```python
from build123d import *

# Parameters (mm, degrees)
F0_W     = 600
F0_H     = 700
F1_DEPTH = 540
F2_W     = 600
F2_H     = 560
F3_DEPTH = 300
F4_W     = 200
F4_H     = 140
F5_DEPTH = 200
F6_W     = 250
F6_H     = 600
F7_DEPTH = 140
F8_R     = 75
F9_DEPTH = 100.001


with BuildPart() as f1:
    # F0 (on Front) → F1 (new body)
    with BuildSketch(Plane.XZ):
        Rectangle(F0_W, F0_H)
    extrude(amount=F1_DEPTH)

    # F2 (on face) → F3 (cut)
    with BuildSketch(Plane.XZ.offset(540)):
        with Locations((0, 70)):
            Rectangle(F2_W, F2_H)
    extrude(amount=-F3_DEPTH, mode=Mode.SUBTRACT)

    # F4 (on face) → F5 (cut)
    with BuildSketch(Plane.XZ.offset(540)):
        with Locations((0, -280)):
            Rectangle(F4_W, F4_H)
    extrude(amount=-F5_DEPTH, mode=Mode.SUBTRACT)

    # F6 (on face) → F7 (cut)
    with BuildSketch(Plane.XZ.offset(240)):
        with BuildLine():
            ThreePointArc((-125, 50), (0, -75), (125, 50))
            Line((125, 50), (-125, 50))
        make_face()
        with Locations((0, 350)):
            Rectangle(F6_W, F6_H)
    extrude(amount=-F7_DEPTH, mode=Mode.SUBTRACT)

    # F8 (on face) → F9 (cut, through all)
    with BuildSketch(Plane.XZ.offset(100)):
        with Locations((0, 100)):
            Circle(F8_R)
    extrude(amount=-F9_DEPTH, mode=Mode.SUBTRACT)


solid = f1.part
```
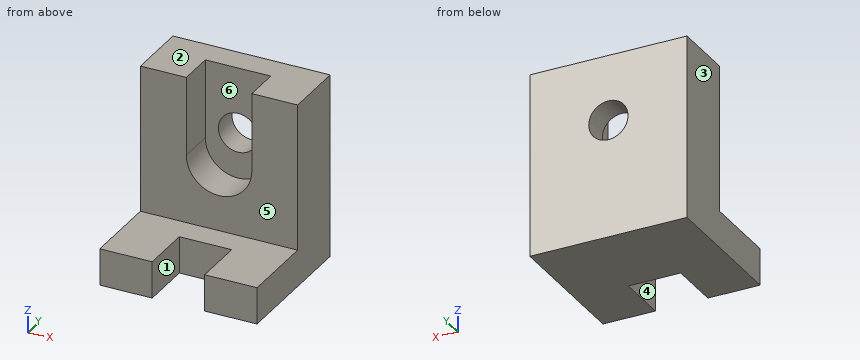
The listing builds one solid part. Answer for the finished solid, in the listing's coordinates (mm). Face numbers are marked on the shaded views. A direction names the side the tool comes from. Coordinates: 2 decimals unless noted, no trailing zeros. Write each loop counter-clockwise with the first axis right and the second up, starting at its lowest first coordinate (ties: lowest second). Pieces come first, ordered by that corner, then holes.
Q1. Section B-B, the plane y = -49 is taken. Write down the section's boundary in (x, z), then the cut area to 3 significant figures.
Returned:
outline: (-300, -350) - (300, -350) - (300, 350) - (-300, 350) - close; hole circle Ø150 at (0, 100)
area: 402,000 mm2
Q2. The mould has two halves that part along X. Classify the marked faces 1, 2 and 3: released by +X, released by -X, zero draft, split by the parting line, or undercut.
Returned:
face 1: undercut
face 2: zero draft
face 3: released by -X
Q3. Which of the six approach directions +Z, -Z, +X, -X, +Y, -Y give full straight-line access (tool end or side, diameter ignored) to the marked faces 4, 5 and 6?
Returned:
face 4: +Z, -Z, -Y
face 5: +Z, +X, -X, -Y
face 6: +Z, -Y
Q4. Find the intervals of material crossed by line 1 along Z through (x, y) = (0, -34); line 2 along Y through (x, z) = (-270, 184); line 3 along Z through (x, y) = (194.5, -493), in increasing order.
Returned:
line 1: z = -350 to 25, 175 to 350
line 2: y = -240 to 0
line 3: z = -350 to -210
Q5. Section A-A, the plane z = 100 is taken. Write down the section's boundary in (x, y), then the cut area to 3 significant figures.
Returned:
outline: (-300, -240) - (-125, -240) - (-125, -100) - (-75, -100) - (-75, 0) - (-300, 0) - close; (75, -100) - (125, -100) - (125, -240) - (300, -240) - (300, 0) - (75, 0) - close
area: 94,000 mm2
Q6. Section C-C, the plane x = 0 is taken. Write down the section's boundary in (y, z), then the cut area to 4 significant figures.
Returned:
outline: (-340, -350) - (0, -350) - (0, 25) - (-100, 25) - (-100, -75) - (-240, -75) - (-240, -210) - (-340, -210) - close; (-100, 175) - (0, 175) - (0, 350) - (-100, 350) - close
area: 107,500 mm2
Q7. Section D-D, the plane z = -280 is taken. Write down the section's boundary in (x, y), then the cut area to 3 significant figures.
Returned:
outline: (-300, -540) - (-100, -540) - (-100, -340) - (100, -340) - (100, -540) - (300, -540) - (300, 0) - (-300, 0) - close
area: 284,000 mm2
Q8. Given P1, Ø5, axis at x = -168.5, z = -135, coming from the -Y side; P2, Ø1.5, axis at x = 167.5, y = -421, coming from the +Z side; P3, Ø6, axis at x = -65.5, y = -109.5, coming from the +Z side, each flat-ended and moving along its own axis, determine where each tip first touches the part or whether it passes through.
Returned:
P1: stops at y = -240
P2: stops at z = -210
P3: stops at z = -54.56
